Drawing for the job (mm, zero at the part's lowest x, y, z). Give positions to 0.01 mm unless a question says otherwise; leave off trailing zeros. Write each loop counter-clockwise with the first axis right and the second up, starting at its lowest first coordinate (ties: lowest second). Pieces come first, ordered by that corner, then holes.
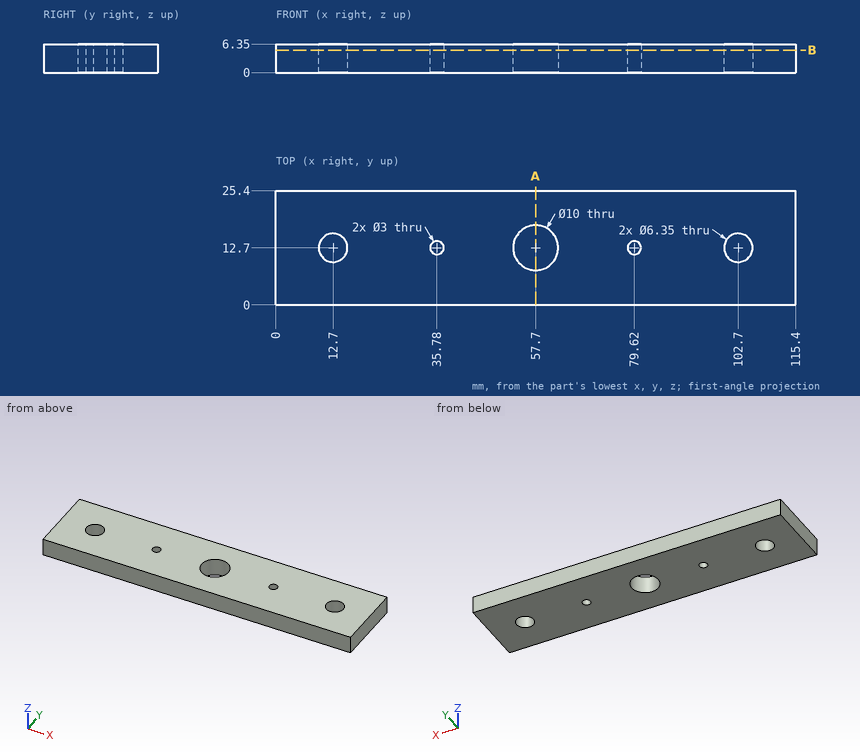
1. Slice it at A-A, the plane x = 57.7. Write the cut outline in (y, z).
Calculated:
outline: (0, 0) - (7.7, 0) - (7.7, 6.35) - (0, 6.35) - close; (17.7, 0) - (25.4, 0) - (25.4, 6.35) - (17.7, 6.35) - close
2. Slice it at B-B, the plane z = 5. State how many separate pieces and enclosed holes the cut face has, and give its area (4 significant figures).
Calculated:
separate pieces: 1
enclosed holes: 5
area: 2,775 mm2
3. Probe probe 1 along X at (y, z) = (14, 1) (1 decimal); probe 2 along Y at (x, z) = (15, 0.5); probe 3 along Y at (x, z) = (13.5, 6.25). List the from-to ranges inside material, lowest first.
Calculated:
probe 1: x = 0 to 9.8, 15.6 to 35, 36.5 to 52.9, 62.5 to 78.9, 80.4 to 99.8, 105.6 to 115.4
probe 2: y = 0 to 10.51, 14.89 to 25.4
probe 3: y = 0 to 9.63, 15.77 to 25.4
